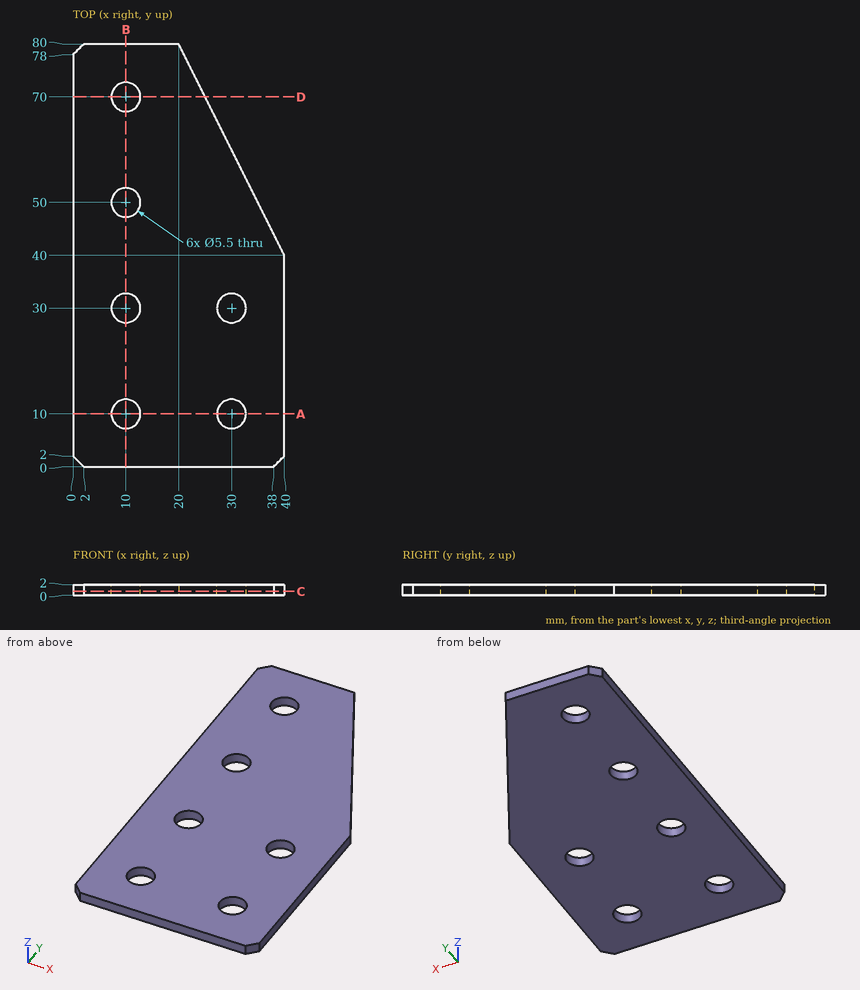
Geometry check sheet. Reference: drawing and pictorial views, mm from the part's lowest x, y, z. Coordinates: 2 decimals unless noted, no trailing zeros. Loops run counter-clockwise (first coordinate to the right, second up) from the corner with the lowest first, then second, coordinate; pieces in that order, holes last. Notation, with made-up numbers: M 10,17 L 56,17 A33 ccw 56,47 Z; hole C 68.5,68 d10. An arc over 180 degrees is marked long. One line per item, written item: value.
1. Section check A-A on y = 10. Record the cut outline in (x, z).
Answers follow:
outline: M 0,0 L 7.25,0 L 7.25,2 L 0,2 Z; M 12.75,0 L 27.25,0 L 27.25,2 L 12.75,2 Z; M 32.75,0 L 40,0 L 40,2 L 32.75,2 Z
2. Gauge pin test, flat end, axial feed: P1, Ø1.5, axis at x = 20.5, y = 20, coming from the -Z side. Record the tip position at first contact, or that the pin passes through.
Answers follow:
P1: z = 0
3. Section check C-C on z = 0.75. Record the cut outline in (x, y), plus the area to 3 significant figures.
Answers follow:
outline: M 0,2 L 2,0 L 38,0 L 40,2 L 40,40 L 20,80 L 2,80 L 0,78 Z; hole C 10,10 d5.5; hole C 10,30 d5.5; hole C 10,50 d5.5; hole C 10,70 d5.5; hole C 30,10 d5.5; hole C 30,30 d5.5
area: 2,650 mm^2
4. Section check D-D on y = 70. Record the cut outline in (x, z), plus the area to 3 significant figures.
Answers follow:
outline: M 0,0 L 7.25,0 L 7.25,2 L 0,2 Z; M 12.75,0 L 25,0 L 25,2 L 12.75,2 Z
area: 39.0 mm^2
5. Material ranges on line 1 along Y through (x, z) = (10, 0.9); line 2 along X through (y, z) = (10, 0.5); line 3 along Y through (x, z) = (8.5, 1.45), recorded low to high. Write a range as from..to.
Answers follow:
line 1: 0..7.25, 12.75..27.25, 32.75..47.25, 52.75..67.25, 72.75..80
line 2: 0..7.25, 12.75..27.25, 32.75..40
line 3: 0..7.7, 12.3..27.7, 32.3..47.7, 52.3..67.7, 72.3..80
6. Section check B-B on x = 10. Record the cut outline in (y, z), plus the area to 3 significant figures.
Answers follow:
outline: M 0,0 L 7.25,0 L 7.25,2 L 0,2 Z; M 12.75,0 L 27.25,0 L 27.25,2 L 12.75,2 Z; M 32.75,0 L 47.25,0 L 47.25,2 L 32.75,2 Z; M 52.75,0 L 67.25,0 L 67.25,2 L 52.75,2 Z; M 72.75,0 L 80,0 L 80,2 L 72.75,2 Z
area: 116 mm^2
